Work out the finished part from the listing and answer in its coordinate system (mm). A direction names the side the tool comes from. Round coordinates to 2 decimals unless told otherwise and drop trailing zeros. Write each loop counter-clockwise with the first axis right and the second up, starting at its lowest first coordinate (ties: lowest second). Pieces come first, ordered by that corner, then holes. Notation, with made-up numbers: (-2, 37.5) - (32, 37.5) arc R18 ccw to (32, 54.5) - close; hole circle Ø3 at (-2, -31.75). An arc over 180 degrees is marked (long way). Answer as a JSON object with one key per item and string values.
```python
from build123d import *

# Parameters (mm, degrees)
F0_W        = 89.5588581535
F0_H        = 165.1
F1_DEPTH    = 6.35
F2_DEPTH    = 25.4
F3_DEPTH    = 50.8
F4_R        = 6.34999
F5_SIZE2    = 7.3323484187
F5_SIZE     = 12.7
F6_C1_SIZE2 = 7.3323484187
F6_C1_SIZE  = 12.7
F6_C2_SIZE2 = 7.3323484187
F6_C2_SIZE  = 12.7
F6_C3_SIZE2 = 12.7
F6_C3_SIZE  = 7.3323484187
F6_C4_SIZE2 = 7.3323484187
F6_C4_SIZE  = 12.7


# Not quite as in the source:
# - a fillet or chamfer is up to 0.001 mm smaller than in the source, because OpenCascade refuses the exact size


with BuildPart() as f1:
    # F0 (on Front) → F1 (new body)
    with BuildSketch(Plane.XZ):
        Rectangle(F0_W, F0_H)
        Polygon((-38.1, 38.1), (-38.1, 76.2), (0, 76.2), (38.1, 76.2), (38.1, -38.1), (38.1, -76.2), (0, -76.2), (-38.1, -76.2), align=None, mode=Mode.SUBTRACT)
    extrude(amount=F1_DEPTH)

    # F0 (on Front) → F2 (join)
    with BuildSketch(Plane.XZ):
        with BuildLine():
            Line((38.1, 76.2), (0, 76.2))
            Line((0, 76.2), (0, 50.8))
            ThreePointArc((0, 50.8), (-3.7197438789, 41.8197438789), (-12.7, 38.1))
            Line((-12.7, 38.1), (-38.1, 38.1))
            Line((-38.1, 38.1), (-38.1, -76.2))
            Line((-38.1, -76.2), (0, -76.2))
            Line((0, -76.2), (0, -50.8))
            ThreePointArc((0, -50.8), (3.7197438789, -41.8197438789), (12.7, -38.1))
            Line((12.7, -38.1), (38.1, -38.1))
            Line((38.1, -38.1), (38.1, 76.2))
        make_face()
    extrude(amount=F2_DEPTH)

    # F0 (on Front) → F3 (join)
    with BuildSketch(Plane.XZ):
        with BuildLine():
            Line((0, 76.2), (-38.1, 76.2))
            Line((-38.1, 76.2), (-38.1, 38.1))
            Line((-38.1, 38.1), (-12.7, 38.1))
            ThreePointArc((-12.7, 38.1), (-3.7197438789, 41.8197438789), (0, 50.8))
            Line((0, 50.8), (0, 76.2))
        make_face()
        with BuildLine():
            Line((38.1, -76.2), (38.1, -38.1))
            Line((38.1, -38.1), (12.7, -38.1))
            ThreePointArc((12.7, -38.1), (3.7197438789, -41.8197438789), (0, -50.8))
            Line((0, -50.8), (0, -76.2))
            Line((0, -76.2), (38.1, -76.2))
        make_face()
    extrude(amount=F3_DEPTH)

    # F4 (radius 6.35 in the source; OpenCascade refuses exactly that, so slightly less here)
    f4_edges = [f1.edges().sort_by_distance(p)[0] for p in [
        (-44.779429, -6.35, 0),
        (0, -6.35, 82.55),
        (0, -6.35, -82.55),
        (44.779429, -6.35, 0),
    ]]
    fillet(f4_edges, radius=F4_R)

    # F5
    f5_edges = [f1.edges().sort_by_distance(p)[0] for p in [
        (-19.05, -25.4, -76.2),
        (38.1, -25.4, 19.05),
        (-38.1, -25.4, -19.05),
        (19.05, -25.4, 76.2),
    ]]
    f5_side = f1.faces().sort_by_distance((0, -25.4, 0))[0]
    chamfer(f5_edges, length=F5_SIZE, length2=F5_SIZE2, reference=f5_side)

    # F6: chamfer of 12.7 x 7.3323484187 on 4 edges, made by hand

    # F6_c1
    f6_c1_edges = [f1.edges().sort_by_distance(p)[0] for p in [
        (-38.1, -50.8, 57.15),
    ]]
    f6_c1_side = f1.faces().sort_by_distance((-38.1, -50.6533530316, 57.15))[0]
    chamfer(f6_c1_edges, length=F6_C1_SIZE, length2=F6_C1_SIZE2, reference=f6_c1_side)

    # F6_c2
    f6_c2_edges = [f1.edges().sort_by_distance(p)[0] for p in [
        (19.05, -50.8, -76.2),
    ]]
    f6_c2_side = f1.faces().sort_by_distance((19.05, -50.6533530316, -76.2))[0]
    chamfer(f6_c2_edges, length=F6_C2_SIZE, length2=F6_C2_SIZE2, reference=f6_c2_side)

    # F6_c3
    f6_c3_edges = [f1.edges().sort_by_distance(p)[0] for p in [
        (-15.3838257906, -50.8, 76.2),
    ]]
    f6_c3_side = f1.faces().sort_by_distance((-15.3838257906, -50.6533530316, 76.2))[0]
    chamfer(f6_c3_edges, length=F6_C3_SIZE, length2=F6_C3_SIZE2, reference=f6_c3_side)

    # F6_c4
    f6_c4_edges = [f1.edges().sort_by_distance(p)[0] for p in [
        (38.1, -50.8, -53.4838257906),
    ]]
    f6_c4_side = f1.faces().sort_by_distance((38.1, -50.6533530316, -53.4838257906))[0]
    chamfer(f6_c4_edges, length=F6_C4_SIZE, length2=F6_C4_SIZE2, reference=f6_c4_side)


solid = f1.part
```
Item 1: A cutting plane is placed at A-A (y = -30.5). Write down the section's boundary in (x, z).
Results found:
{"outline": "(-38.1, 38.1) - (-12.7, 38.1) arc R12.7 ccw to (0, 50.8) - (0, 76.2) - (-38.1, 76.2) - close; (0, -76.2) - (38.1, -76.2) - (38.1, -38.1) - (12.7, -38.1) arc R12.7 ccw to (0, -50.8) - close"}
Item 2: Each of these flat-tipped pins is pushed along its axis until it touches: P1, Ø6, axis at x = -33, z = -9.5, coming from the +Y side; P2, Ø18.5, axis at x = -6, y = -25.5, coming from the +Z side; P3, Ø5, axis at x = -7, z = -61.5, coming from the -Y side; P4, Ø20.5, axis at x = -25.5, y = -37, coming from the -Z side. Where does it stop, or does it pass through?
Results found:
{"P1": "y = 0", "P2": "z = 76.2", "P3": "y = -25.4", "P4": "z = 38.1"}
Item 3: Consider line 1 along Y through (x, z) = (-19, -25); line 2 along Y through (x, z) = (-38.5, 64.5); line 3 along Z through (x, y) = (21.5, -31). Determine where each line is inside the solid, lowest interval first.
Results found:
{"line 1": "-25.4 to 0", "line 2": "-6.35 to 0", "line 3": "-76.2 to -38.1"}
Item 4: For faces 1 (the flat face through (-8, -21, 76.2)), 2 (the flat face through (38.1, -15, -18)), 3 (the flat face through (0, -25.4, 1)), determine the directions among +Z, -Z, +X, -X, +Y, -Y from which every point of the face is accessible in a straight line to the end or side of a thin tool.
Results found:
{"face 1": "+Z, +X, -X, -Y", "face 2": "+Z, -Z, +X, -Y", "face 3": "-Y"}
Item 5: A cutting plane is placed at D-D (y = -8). Write down the section's boundary in (x, z), and give its area (3 significant figures).
Results found:
{"outline": "(-38.1, -76.2) - (38.1, -76.2) - (38.1, 76.2) - (-38.1, 76.2) - close", "area": "11,600 mm²"}
